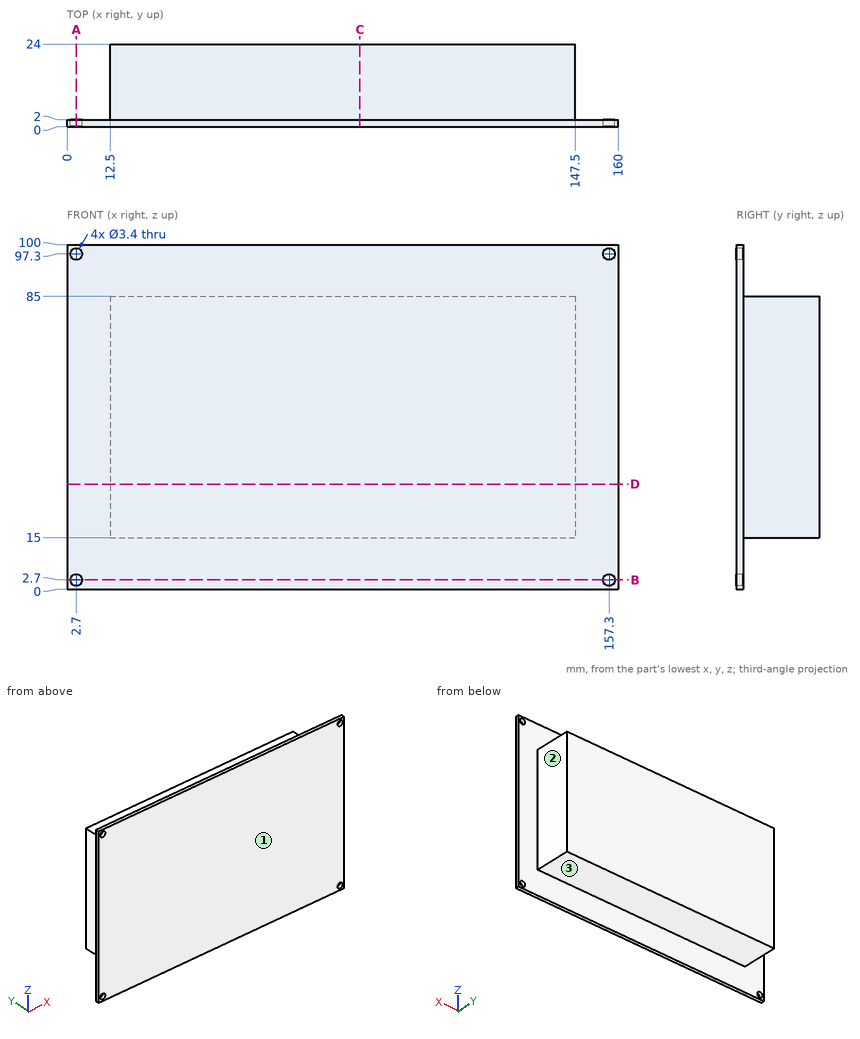
Answer from the drawing. Dimensions are ordinates in mm from the lowest x, y and z of the part. A direction names the side the tool comes from. Give positions to 0.01 mm unless a question says otherwise; leave off trailing zeros. Loops run counter-clockwise (first coordinate to the right, second up) from the corner with the lowest first, then second, coordinate; pieces in that order, holes last. Notation, with made-up numbers: (89.25, 32) - (111.25, 32) arc R22 ccw to (111.25, 46) - close; hole circle Ø11 at (57.5, -30). An arc over 180 degrees is marked (long way). Write each question's results on one line, items separated by ' | '.
1. Consider probe 1 along Z at (x, y) = (157.3, 0.5); probe 2 along X at (y, z) = (0.65, 97.3); probe 3 along Z at (x, y) = (122, 11). Determine where each line is inside the solid, lowest interval first. Write a range as from..to.
Resolved:
probe 1: z = 0..1, 4.4..95.6, 99..100 | probe 2: x = 0..1, 4.4..155.6, 159..160 | probe 3: z = 15..85
2. Find section D-D, the plane z = 30.5. Write down the section's boundary in (x, y).
Resolved:
outline: (0, 0) - (160, 0) - (160, 2) - (147.5, 2) - (147.5, 24) - (12.5, 24) - (12.5, 2) - (0, 2) - close
3. Which of the six approach directions +Z, -Z, +X, -X, +Y, -Y give full straight-line access (tool end or side, diameter ignored) to the marked faces 1, 2 and 3?
Resolved:
face 1: +Z, -Z, +X, -X, -Y | face 2: +Z, -Z, +X, +Y | face 3: -Z, +X, -X, +Y
4. Find section C-C, the plane x = 85. Write down the section's boundary in (y, z), then the cut area to 3 significant figures.
Resolved:
outline: (0, 0) - (2, 0) - (2, 15) - (24, 15) - (24, 85) - (2, 85) - (2, 100) - (0, 100) - close | area: 1,740 mm^2
5. Find section B-B, the plane z = 2.7. Write down the section's boundary in (x, y), then the cut area to 3 significant figures.
Resolved:
outline: (0, 0) - (1, 0) - (1, 2) - (0, 2) - close; (4.4, 0) - (155.6, 0) - (155.6, 2) - (4.4, 2) - close; (159, 0) - (160, 0) - (160, 2) - (159, 2) - close | area: 306 mm^2
6. Find section A-A, the plane x = 2.7. Write down the section's boundary in (y, z), then the cut area to 3 significant figures.
Resolved:
outline: (0, 0) - (2, 0) - (2, 1) - (0, 1) - close; (0, 4.4) - (2, 4.4) - (2, 95.6) - (0, 95.6) - close; (0, 99) - (2, 99) - (2, 100) - (0, 100) - close | area: 186 mm^2
7. Flat-ended cylindrical pins translate along their axes: P1, Ø10, axis at x = 119.5, y = 17.5, coming from the +Z side; P2, Ø2, axis at x = 74, y = 8, coming from the -Z side; P3, Ø11, axis at y = 11, z = 57, coming from the +X side; P4, Ø3, axis at x = 2.7, z = 97.3, coming from the -Y side. Find the tip coordinate at first contact, or state that the pin passes through.
Resolved:
P1: stops at z = 85 | P2: stops at z = 15 | P3: stops at x = 147.5 | P4: passes through
